```python
from build123d import *

# Parameters (mm, degrees)
SKETCH_1_W               = 60
SKETCH_1_H               = 40
EXTRUDE_1_DEPTH          = 40
SKETCH_2_W               = 40
SKETCH_2_H               = 6
CUT_EXTRUDE_1_DEPTH      = 83.462112512
CUT_EXTRUDE_2_DEPTH      = 76.498344353
CUT_EXTRUDE_2_DEPTH_BACK = 76.498344353
SKETCH_6_W               = 29.277204284
SKETCH_6_H               = 28
EXTRUDE_2_REACH          = 84.462
SKETCH_7_W               = 28
SKETCH_7_H               = 8
EXTRUDE_4_DEPTH          = 5
SKETCH_12_R              = 5
CUT_EXTRUDE_4_DEPTH      = 78.356318423
FILLET_1_R               = 8
SKETCH_14_R              = 6
CUT_EXTRUDE_5_DEPTH      = 75.833147735


with BuildPart() as part:
    # 草图1 → 凸台-拉伸1 (new body)
    with BuildSketch(Plane(origin=(0, 0, 0), x_dir=(1, 0, 0), z_dir=(0, 1, 0))):
        with Locations((30, -20)):
            Rectangle(SKETCH_1_W, SKETCH_1_H)
    extrude(amount=EXTRUDE_1_DEPTH)

    # 草图2 → 切除-拉伸1 (cut, through all)
    with BuildSketch(Plane(origin=(0, 40, 0), x_dir=(1, 0, 0), z_dir=(0, 1, 0))):
        with Locations((30, -3)):
            Rectangle(SKETCH_2_W, SKETCH_2_H)
    extrude(amount=-CUT_EXTRUDE_1_DEPTH, mode=Mode.SUBTRACT)

    # 草图6 → 切除-拉伸2 (cut, two sides: drawn at the far end of the back side and taken through both)
    with BuildSketch(Plane.ZY.offset(-50).offset(-CUT_EXTRUDE_2_DEPTH_BACK)):
        with Locations((25.361397858, 26)):
            Rectangle(SKETCH_6_W, SKETCH_6_H)
    extrude(amount=CUT_EXTRUDE_2_DEPTH + CUT_EXTRUDE_2_DEPTH_BACK, mode=Mode.SUBTRACT)

    # 草图7 → 凸台-拉伸2 (add, up to next)
    with BuildSketch(Plane.XY.offset(40), mode=Mode.PRIVATE) as extrude_2_sk1:
        with Locations((30, 16)):
            Rectangle(SKETCH_7_W, SKETCH_7_H)
    extrude_2_tool1 = extrude(extrude_2_sk1.sketch, amount=-EXTRUDE_2_REACH, mode=Mode.PRIVATE) - part.part
    add(extrude_2_tool1.solids().sort_by_distance((30, 16, 40))[0])

    # 草图8 → 凸台-拉伸4 (add)
    with BuildSketch(Plane(origin=(0, 20, 0), x_dir=(1, 0, 0), z_dir=(0, 1, 0))):
        with BuildLine():
            ThreePointArc((24, -39.980933727), (30, -33.980933727), (36, -39.980933727))
            Line((36, -39.980933727), (42, -39.980933727))
            ThreePointArc((42, -39.980933727), (30, -27.980933727), (18, -39.980933727))
            Line((18, -39.980933727), (24, -39.980933727))
        make_face()
    extrude(amount=EXTRUDE_4_DEPTH)

    # 草图12 → 切除-拉伸4 (cut, through all)
    with BuildSketch(Plane(origin=(0, 12, 0), x_dir=(1, 0, 0), z_dir=(0, 1, 0))):
        with Locations(Location((8, -30.722795716, 0), (0, 0, 270))):
            Circle(SKETCH_12_R)
        with Locations(Location((52, -30.722795716, 0), (0, 0, 270))):
            Circle(SKETCH_12_R)
    extrude(amount=-CUT_EXTRUDE_4_DEPTH, mode=Mode.SUBTRACT)

    # 圆角1
    fillet_1_edges = [part.edges().sort_by_distance(p)[0] for p in [
        (60, 6, 40),
        (0, 6, 40),
    ]]
    fillet(fillet_1_edges, radius=FILLET_1_R)

    # 草图14 → 切除-拉伸5 (cut, through all)
    with BuildSketch(Plane(origin=(0, 20, 0), x_dir=(1, 0, 0), z_dir=(0, 1, 0))):
        with Locations((30, -40)):
            Circle(SKETCH_14_R)
    extrude(amount=-CUT_EXTRUDE_5_DEPTH, mode=Mode.SUBTRACT)


solid = part.part
```
Work out the finished part from the listing and answer in its coordinate system (mm). A direction names the side the tool comes from. Round coordinates to 2 decimals unless told otherwise and drop trailing zeros. Loops run counter-clockwise (first coordinate to the right, second up) from the corner with the lowest first, then second, coordinate; pieces in that order, holes last. Notation, with made-up numbers: M 45,52.5 L 85,52.5 A32 cw 85,79.5 Z; hole C -17.5,-12.75 d10. An arc over 180 degrees is marked long. One line per question, with ' | ' between items.
Q1. Each of these flat-tipped pins is pushed along its axis until it touches: pin 1 Ø13 at (x, z) = (29.5, 33) entering from +Y; pin 2 Ø5 at (x, z) = (12, 23.5) entering from +Y; pin 3 Ø4 at (y, z) = (14.5, 18.5) entering from +X. Where does it stop, or does it pass through?
Conclusion:
pin 1: stops at y = 25 | pin 2: stops at y = 12 | pin 3: stops at x = 44
Q2. A tool of negligible diameter and unlimited length cuts with its end or side. For faces 4 (the cylindrical face through (30.264, 22.465, 27.984)), 5 (the flat face through (16, 16, 26)), 6 (the flat face through (30, 20, 6)), 7 (the flat face through (30, 25, 33)), from which of +Z, -Z, +X, -X, +Y, -Y can it reach the whole face along a straight path? Write none if from no direction.
Conclusion:
face 4: +Y | face 5: +Z, -X, +Y | face 6: -Z, +Y, -Y | face 7: +Z, +X, -X, +Y
Q3. Find section A-A, the plane z = 4. Give the vertices of the cut face in (x, y), then the cut area to 3 significant figures.
Conclusion:
outline: M 0,0 L 10,0 L 10,40 L 0,40 Z; M 50,0 L 60,0 L 60,40 L 50,40 Z | area: 800 mm2
Q4. The mould has two halves that part along X. Classify faces 1 (the cylindrical face through (56.957, 6.084, 30.072)), 2 (the flat face through (30, 0, 20)), 3 (the flat face through (44, 16, 26)): +X half, -X half, draft (parallel to the pull), parting line (faces both ways), or undercut.
Conclusion:
face 1: undercut | face 2: draft | face 3: +X half
Q5. Find section C-C, the plane z = 20. Give the vertices of the cut face in (x, y).
Conclusion:
outline: M 0,0 L 60,0 L 60,12 L 44,12 L 44,20 L 16,20 L 16,12 L 0,12 Z
Q6. Find section D-D, the plane x = 46. Give the vertices of the cut face in (y, z), then the cut area to 3 significant figures.
Conclusion:
outline: M 0,6 L 40,6 L 40,10.72 L 12,10.72 L 12,40 L 0,40 Z | area: 540 mm2
Q7. Find section B-B, the plane y = 3.5. Give the vertices of the cut face in (x, z).
Conclusion:
outline: M 0,0 L 10,0 L 10,6 L 50,6 L 50,0 L 60,0 L 60,32 A8 ccw 52,40 L 36,40 A6 cw 24,40 L 8,40 A8 ccw 0,32 Z; hole C 8,30.72 d10; hole C 52,30.72 d10
Q8. Consider line 1 along Z through (x, y) = (43.5, 11.5); line 2 along Y through (x, z) = (10, 20); line 3 along Z through (x, y) = (7.5, 9.5). Determine where each line is inside the solid, lowest interval first. Write a range as from..to.
Conclusion:
line 1: z = 6..40 | line 2: y = 0..12 | line 3: z = 0..25.75, 35.7..39.98
